Source: CAD feature listing. Evaluate the final solid. Frame: model axes, mm. A direction names the side the tool comes from. Coordinates: 2 decimals unless noted, no trailing zeros. Order: outer loops, then holes, each group sorted by start corner. A loop starts at its lowest first (then second) coordinate and runs counter-clockwise, first axis right, second up.
```python
from build123d import *

# Parameters (mm, degrees)
EXTRUDE_1_DEPTH     = 23
SKETCH_2_R          = 4.25
CUT_EXTRUDE_1_DEPTH = 5
SKETCH_3_R          = 4.25
CUT_EXTRUDE_2_DEPTH = 5
FILLET_1_R          = 4
FILLET_2_R          = 1


with BuildPart() as part:
    # Эскиз1 → Бобышка-Вытянуть1 (new body, symmetric)
    with BuildSketch(Plane.XY):
        Polygon((0, 0), (42.426406871, 42.426406871), (45.961940777, 38.890872965), (20.266663343, 13.195595531), (23.661390163, 5), (60, 5), (60, 0), align=None)
        Polygon((17.142135624, 12.899494937), (21.242640687, 3), (7.242640687, 3), align=None, mode=Mode.SUBTRACT)
    extrude(amount=EXTRUDE_1_DEPTH, both=True)

    # Эскиз2 → Вырез-Вытянуть1 (cut)
    with BuildSketch(Plane(origin=(0, 0, 0), x_dir=(0, 0, 1), z_dir=(-0.707106781, 0.707106781, 0))):
        with Locations(Location((0, 45, 0), (0, 0, 270))):  # turned: the seam where the file's is
            Circle(SKETCH_2_R)
    extrude(amount=-CUT_EXTRUDE_1_DEPTH, mode=Mode.SUBTRACT)

    # Эскиз3 → Вырез-Вытянуть2 (cut)
    with BuildSketch(Plane.XZ):
        with Locations(Location((45, 0, 0), (0, 0, 270))):  # turned: the seam where the file's is
            Circle(SKETCH_3_R)
    extrude(amount=-CUT_EXTRUDE_2_DEPTH, mode=Mode.SUBTRACT)

    # Скругление1
    fillet_1_edges = [part.edges().sort_by_distance(p)[0] for p in [
        (45.961940777, 38.890872965, 0),
        (60, 5, 0),
    ]]
    fillet(fillet_1_edges, radius=FILLET_1_R)

    # Скругление2
    fillet_2_edges = [part.edges().sort_by_distance(p)[0] for p in [
        (17.142135624, 12.899494937, 0),
        (7.242640687, 3, 0),
        (21.242640687, 3, 0),
    ]]
    fillet(fillet_2_edges, radius=FILLET_2_R)


solid = part.part
```
1. Pin query (flat end, axial travel): P1, Ø10, axis at y = 38, z = 1, coming from the +X side; P2, Ø7.5, axis at x = 45, z = 0, coming from the -Y side; P3, Ø3, axis at y = 25.5, z = 0, coming from the -X side; P4, Ø12, axis at x = 50.5, y = 30, coming from the +Z side. Return the tip coordinate at first contact, or that it passes through.
Findings:
P1: stops at x = 44.31
P2: stops at y = 34.18
P3: stops at x = 24
P4: passes through
2. Section query D-D on x = 26.5. Return loops of the section in (y, z), plus the area to 3 significant figures.
Findings:
outline: (0, -23) - (5, -23) - (5, 23) - (0, 23) - close; (19.43, -23) - (26.5, -23) - (26.5, 23) - (19.43, 23) - close
area: 555 mm2
3. Draft query along Y for faces 4 (the face through (40.85, 2.46, 0.92)), 5 (the face through (19.17, 8, 0.32)), 6 (the face through (36.565, 33.079, 0.187)), 7 (the face through (58.859, 3.797, 0.322)). Return one class per face: released by +Y, released by -Y, zero draft, split by the parting line, or undercut.
Findings:
face 4: zero draft
face 5: undercut
face 6: undercut
face 7: released by +Y
4. Access query for faces 1 (the face through (30, 0, 0)), 2 (the face through (15, 3, 0)), 3 (the face through (31.86, 24.79, 0.32)). Directions: +Z, -Z, +X, -X, +Y, -Y. A direction counts if a zero-diameter tool reaches every point of the face in a straight line with its end or side. Return the directions, or none.
Findings:
face 1: +Z, -Z, +X, -X, -Y
face 2: +Z, -Z
face 3: +Z, -Z, +X
5. Section query B-B on z = 12. Return loops of the section in (x, y), plus the area to 3 significant figures.
Findings:
outline: (0, 0) - (60, 0) - (60, 1) arc R4 ccw to (56, 5) - (23.66, 5) - (20.27, 13.2) - (43.13, 36.06) arc R4 ccw to (43.13, 41.72) - (42.43, 42.43) - close; hole (8.95, 4.71) arc R1 ccw to (9.66, 3) - (19.75, 3) arc R1 ccw to (20.67, 4.38) - (17.71, 11.52) arc R1 ccw to (16.08, 11.84) - close
area: 513 mm2
6. Section query C-C on z = 0. Return loops of the section in (x, y) (3 decimals).
Findings:
outline: (0, 0) - (40.75, 0) - (40.75, 5) - (23.661, 5) - (20.267, 13.196) - (32.35, 25.279) - (28.815, 28.815) - close; (34.825, 34.825) - (38.361, 31.289) - (43.134, 36.062) arc R4 ccw to (43.134, 41.719) - (42.426, 42.426) - close; (49.25, 0) - (60, 0) - (60, 1) arc R4 ccw to (56, 5) - (49.25, 5) - close; hole (8.95, 4.707) arc R1 ccw to (9.657, 3) - (19.746, 3) arc R1 ccw to (20.67, 4.383) - (17.715, 11.517) arc R1 ccw to (16.084, 11.841) - close
7. Section query A-A on x = 45. Return loops of the section in (y, z).
Findings:
outline: (0, -23) - (5, -23) - (5, -4.25) - (0, -4.25) - close; (0, 4.25) - (5, 4.25) - (5, 23) - (0, 23) - close
8. Ray query, line 1 (X direction, y = 3.2, z = 0); line 2 (Y direction, x = 48, z = 10.5); line 3 (X direction, y = 3.1, z = 0). Return the intervals inside material, ascending.
Findings:
line 1: x = 3.2 to 9.06, 20.35 to 40.75, 49.25 to 59.34
line 2: y = 0 to 5
line 3: x = 3.1 to 9.22, 20.18 to 40.75, 49.25 to 59.4
